Geometry check sheet. Reference: drawing and pictorial views, mm from the part's lowest x, y, z. A direction names the side the tool comes from. Round coordinates to 2 decimals unless told otherwise and drop trailing zeros. Write each loop counter-clockwise with the first axis right and the second up, starting at its lowest first coordinate (ties: lowest second). Pieces come first, ordered by that corner, then holes. Notation, with made-up numbers: (18.25, 9.25) - (59.25, 9.25) arc R33 cw to (59.25, 43.25) - close; hole circle Ø7 at (13.5, -18.75). An arc over 180 degrees is marked (long way). Return JSON: item names as keys, results as strings.
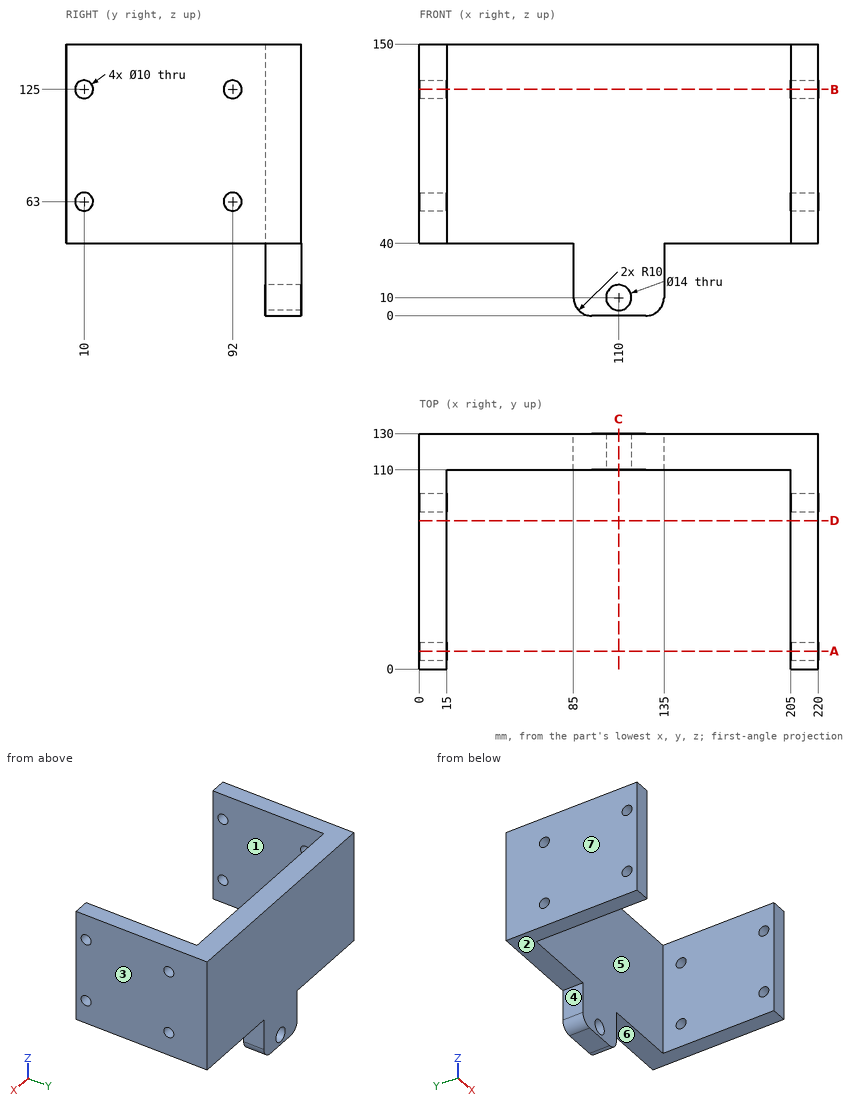
(1) Gauge pin test, flat ends, axial feed: pin 1 (10 mm diameter, centred on y = 122, z = 31.5, fed in from -X); pin 2 (4 mm diameter, centred on x = 29.5, z = 103, fed in from -Y). Record the tip position at first contact, or that the pin passes through.
Response values:
{"pin 1": "stops at x = 85", "pin 2": "stops at y = 110"}
(2) Section check C-C, the plane x = 110. Enter the section's corners in (y, z).
Response values:
{"outline": "(110, 0) - (130, 0) - (130, 3) - (110, 3) - close; (110, 17) - (130, 17) - (130, 150) - (110, 150) - close"}
(3) Section check D-D, the plane y = 82. Enter the section's corners in (x, z).
Response values:
{"outline": "(0, 40) - (15, 40) - (15, 150) - (0, 150) - close; (205, 40) - (220, 40) - (220, 150) - (205, 150) - close"}
(4) Release check for a two-part mould opening along X. For the marked faces 1, 2, 3 and 4 record: pulls with the +X half, pulls with the -X half, needs draft (parallel to the pull), parting line crosses it, or undercut.
Response values:
{"face 1": "undercut", "face 2": "needs draft", "face 3": "pulls with the +X half", "face 4": "pulls with the -X half"}
(5) Section check A-A, the plane y = 10. Enter the section's corners in (x, z), plus the area to 3 significant figures.
Response values:
{"outline": "(0, 40) - (15, 40) - (15, 58) - (0, 58) - close; (0, 68) - (15, 68) - (15, 120) - (0, 120) - close; (0, 130) - (15, 130) - (15, 150) - (0, 150) - close; (205, 40) - (220, 40) - (220, 58) - (205, 58) - close; (205, 68) - (220, 68) - (220, 120) - (205, 120) - close; (205, 130) - (220, 130) - (220, 150) - (205, 150) - close", "area": "2,700 mm^2"}
(6) Material ranges on line 1 along Y through (x, z) = (208, 125); line 2 along X through (y, z) = (96, 132.5); line 3 along Y through (x, z) = (17, 125.5), recorded low to high. Write a range as [from, to].
Response values:
{"line 1": "y = [0, 5], [15, 87], [97, 130]", "line 2": "x = [0, 15], [205, 220]", "line 3": "y = [110, 130]"}
(7) Access from +Z, -Z, +X, -X, +Y, -Y to the whole of each face (thin tool, end or side, straight path). Record for the marked faces 5, 6 and 7.
Response values:
{"face 5": "+Z, -Z, -Y", "face 6": "-Z, +X, +Y, -Y", "face 7": "+Z, -Z, -X, +Y, -Y"}
(8) Section check B-B, the plane z = 125. Enter the section's corners in (x, y).
Response values:
{"outline": "(0, 0) - (15, 0) - (15, 5) - (0, 5) - close; (0, 15) - (15, 15) - (15, 87) - (0, 87) - close; (0, 97) - (15, 97) - (15, 110) - (205, 110) - (205, 97) - (220, 97) - (220, 130) - (0, 130) - close; (205, 0) - (220, 0) - (220, 5) - (205, 5) - close; (205, 15) - (220, 15) - (220, 87) - (205, 87) - close"}
